```python
from build123d import *

# Parameters (mm, degrees)
F0_R     = 47.5
F0_R_2   = 45.5
F1_DEPTH = 3
F2_W     = 100
F2_H     = 100
F2_R     = 45.5
F3_DEPTH = 2


with BuildPart() as f1:
    # F0 (on Top) → F1 (new body)
    with BuildSketch(Plane.XY):
        Circle(F0_R)
        Circle(F0_R_2, mode=Mode.SUBTRACT)
    extrude(amount=F1_DEPTH)

    # F2 (on Top) → F3 (join)
    with BuildSketch(Plane.XY):
        Rectangle(F2_W, F2_H)
        Circle(F2_R, mode=Mode.SUBTRACT)
    extrude(amount=-F3_DEPTH)


solid = f1.part
```
Geometry: final body of the model. Coordinates: model frame, mm. A direction names the side the tool comes from. Coordinates: 2 decimals unless noted, no trailing zeros. Order: outer loops, then holes, each group sorted by start corner. A loop starts at its lowest first (then second) coordinate and runs counter-clockwise, first axis right, second up. Notation, with made-up numbers: (13, 38) -> (61, 38) arc R28 ccw to (61, 64) -> close; hole circle Ø7 at (58.25, 76.5). An arc over 180 degrees is marked (long way). Write item = value, one per line.
(1) Access query for faces 1 (the flat face through (0, -46, 3)), 2 (the flat face through (-29.9, 37.3, 0)). Directions: +Z, -Z, +X, -X, +Y, -Y. A direction counts if a zero-diameter tool reaches every point of the face in a straight line with its end or side. Return the directions, or none.
Solved:
face_1 = +Z, +X, -X, +Y, -Y
face_2 = +Z
(2) Line query: line 1 (Y direction, x = 0, z = -0.8); line 2 (Z direction, x = 42, y = -35); line 3 (Y direction, x = 19.5, z = 0.8). Output: solid intervals per line, ascending.
Solved:
line_1 = -50 to -45.5, 45.5 to 50
line_2 = -2 to 0
line_3 = -43.31 to -41.11, 41.11 to 43.31
(3) Pin query (flat end, axial travel): pin 1 Ø1 at (x, z) = (-15, 1.5) entering from -Y. Return the tip coordinate at first contact, or that it passes through.
Solved:
pin_1 = -45.23
(4) Cut plane C-C on z = 1.35. Return loops of the section in (x, y).
Solved:
outline = circle Ø95 at (0, 0); hole circle Ø91 at (0, 0)
(5) Cut plane A-A on x = 0. Return loops of the section in (y, z).
Solved:
outline = (-50, -2) -> (-45.5, -2) -> (-45.5, 3) -> (-47.5, 3) -> (-47.5, 0) -> (-50, 0) -> close; (45.5, -2) -> (50, -2) -> (50, 0) -> (47.5, 0) -> (47.5, 3) -> (45.5, 3) -> close
